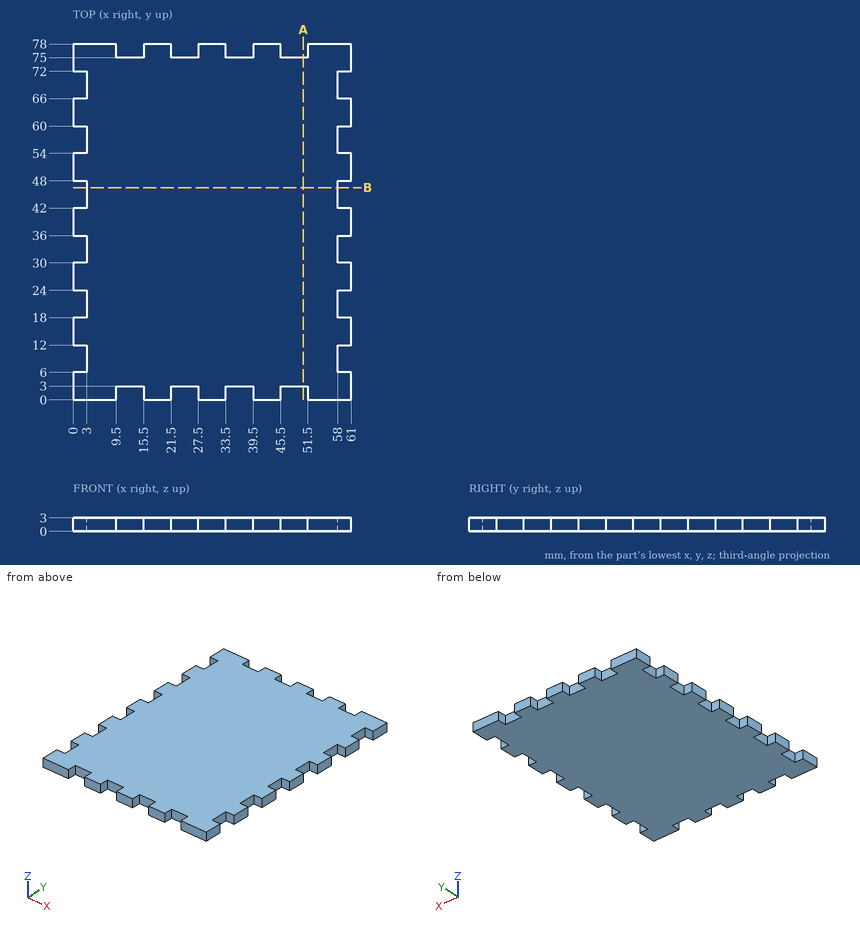
Geometry check sheet. Reference: drawing and pictorial views, mm from the part's lowest x, y, z. Round coordinates to 2 decimals unless told otherwise and drop trailing zeros. Write each loop counter-clockwise with the first axis right and the second up, starting at its lowest first coordinate (ties: lowest second). Pieces come first, ordered by that corner, then holes.
Item 1: Section check B-B (y = 46.5). Record the boundary of the cut face in (x, z).
Determined:
outline: (3, 0) - (58, 0) - (58, 3) - (3, 3) - close
Item 2: Section check A-A (x = 50.5). Record the boundary of the cut face in (y, z).
Determined:
outline: (3, 0) - (75, 0) - (75, 3) - (3, 3) - close
Item 3: Material ranges on line 1 along Y through (x, z) = (11.5, 2.5); line 2 along X through (y, z) = (34, 0.5), recorded low to high.
Determined:
line 1: y = 3 to 75
line 2: x = 3 to 58
Item 4: Go/stop test with flat-tipped pins: pin 1 Ø1.5 at (y, z) = (9, 1.5) entering from -X; pin 2 Ø1.5 at (y, z) = (8, 1) entering from +X; pin 3 Ø1 at (x, z) = (35.5, 2.5) entering from +Y. Record where each tip stops, or that it passes through.
Determined:
pin 1: stops at x = 3
pin 2: stops at x = 58
pin 3: stops at y = 75
